Input: part model. Units: mm. Frame: model coordinates. Face numbers are marked on the shaded views. Give positions to 0.01 mm unless a question says otherwise; leave off trailing zeros. Order: outer loops, then holes, each group sorted by start corner. A loop starts at its lowest first (then second) coordinate and runs counter-clockwise, first axis right, second up. Notation, with made-up numbers: (74, 56) -> (125, 56) arc R30 cw to (125, 92) -> close; hole circle Ø4 at (67, 86.5). An arc over 180 degrees is marked (long way). Use a Markdown table: item, result. Add a question column.
from build123d import *

# Parameters (mm, degrees)
F0_R     = 14.2875
F1_DEPTH = 25.4
F2_DEPTH = 50.8


with BuildPart() as f1:
    # F0 (on Front) → F1 (new body)
    with BuildSketch(Plane.XZ):
        with BuildLine():
            Line((9.5121844836, 26.9452959039), (0, 28.575))
            ThreePointArc((0, 28.575), (-28.575, 0), (0, -28.575))
            Line((0, -28.575), (9.5121844836, -26.9452959039))
            ThreePointArc((9.5121844836, -26.9452959039), (23.3274655355, -16.5033322905), (28.575, 0))
            ThreePointArc((28.575, 0), (23.3274655355, 16.5033322905), (9.5121844836, 26.9452959039))
        make_face()
        with BuildLine():
            ThreePointArc((-14.6329037383, 4.7625), (0, 15.3884137605), (14.6329037383, 4.7625))
            Line((14.6329037383, 4.7625), (19.05, 4.7625))
            Line((19.05, 4.7625), (19.05, -4.7625))
            Line((19.05, -4.7625), (14.6329037383, -4.7625))
            ThreePointArc((14.6329037383, -4.7625), (0, -15.3884137605), (-14.6329037383, -4.7625))
            Line((-14.6329037383, -4.7625), (-19.05, -4.7625))
            Line((-19.05, -4.7625), (-19.05, 4.7625))
            Line((-19.05, 4.7625), (-14.6329037383, 4.7625))
        make_face(mode=Mode.SUBTRACT)
        with BuildLine():
            Line((57.1919272622, 18.7764181619), (9.5121844836, 26.9452959039))
            ThreePointArc((9.5121844836, 26.9452959039), (23.3274655355, 16.5033322905), (28.575, 0))
            ThreePointArc((28.575, 0), (23.3274655355, -16.5033322905), (9.5121844836, -26.9452959039))
            Line((9.5121844836, -26.9452959039), (57.1919272622, -18.7764181619))
            ThreePointArc((57.1919272622, -18.7764181619), (34.925, 0), (57.1919272622, 18.7764181619))
        make_face()
        with BuildLine():
            ThreePointArc((73.025, 0), (68.5383952831, 12.2804730295), (57.1919272622, 18.7764181619))
            ThreePointArc((57.1919272622, 18.7764181619), (34.925, 0), (57.1919272622, -18.7764181619))
            ThreePointArc((57.1919272622, -18.7764181619), (68.5383952831, -12.2804730295), (73.025, 0))
        make_face()
        with Locations((53.975, 0)):
            Circle(F0_R, mode=Mode.SUBTRACT)
        with BuildLine():
            ThreePointArc((-14.6329037383, -4.7625), (-15.3884137605, 0), (-14.6329037383, 4.7625))
            Line((-14.6329037383, 4.7625), (-19.05, 4.7625))
            Line((-19.05, 4.7625), (-19.05, -4.7625))
            Line((-19.05, -4.7625), (-14.6329037383, -4.7625))
        make_face()
    extrude(amount=F1_DEPTH)

    # F0 (on Front) → F2 (join)
    with BuildSketch(Plane.XZ):
        with BuildLine():
            Line((9.5121844836, 26.9452959039), (0, 28.575))
            ThreePointArc((0, 28.575), (-28.575, 0), (0, -28.575))
            Line((0, -28.575), (9.5121844836, -26.9452959039))
            ThreePointArc((9.5121844836, -26.9452959039), (23.3274655355, -16.5033322905), (28.575, 0))
            ThreePointArc((28.575, 0), (23.3274655355, 16.5033322905), (9.5121844836, 26.9452959039))
        make_face()
        with BuildLine():
            ThreePointArc((-14.6329037383, 4.7625), (0, 15.3884137605), (14.6329037383, 4.7625))
            Line((14.6329037383, 4.7625), (19.05, 4.7625))
            Line((19.05, 4.7625), (19.05, -4.7625))
            Line((19.05, -4.7625), (14.6329037383, -4.7625))
            ThreePointArc((14.6329037383, -4.7625), (0, -15.3884137605), (-14.6329037383, -4.7625))
            Line((-14.6329037383, -4.7625), (-19.05, -4.7625))
            Line((-19.05, -4.7625), (-19.05, 4.7625))
            Line((-19.05, 4.7625), (-14.6329037383, 4.7625))
        make_face(mode=Mode.SUBTRACT)
        with BuildLine():
            ThreePointArc((-14.6329037383, -4.7625), (-15.3884137605, 0), (-14.6329037383, 4.7625))
            Line((-14.6329037383, 4.7625), (-19.05, 4.7625))
            Line((-19.05, 4.7625), (-19.05, -4.7625))
            Line((-19.05, -4.7625), (-14.6329037383, -4.7625))
        make_face()
    extrude(amount=F2_DEPTH)


solid = f1.part
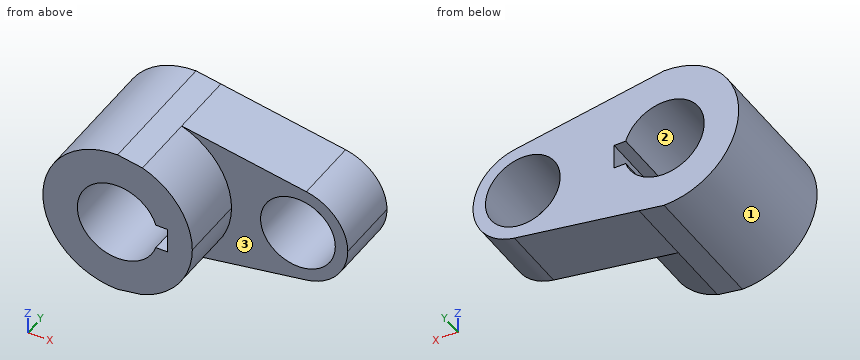
Q1. Section query B-B (z = -7.5). Return loops of the section in (x, y), plus the area to 3 significant figures.
Q2. First-contact query: pin 1 (3.5 mm diameter, centred on x = 16.5, y = -33, fed in from +Z); pin 2 (10.5 mm diameter, centred on y = -13.5, z = -1.5, fed in from -X) (3 decimals); pin 3 (3 mm diameter, centred on x = 7.5, z = -11.5, fed in from +Y); pin 4 (16 mm diameter, centred on x = 46.5, z = 7, fed in from -Y). Flat tips, straight axial feed; report the tip coordinate or a pass-through.
Q3. Ray query, line 1 (X direction, y = -10.5, z = -8.5); line 2 (X direction, y = -11.5, z = -3.5); line 3 (Y direction, x = 44.5, z = -14). Return the intervals inside material, ascending.
Q4. Section query D-D (x = 52). Return loops of the section in (y, z).
Q5. Draft query along X for the marked faces 1, 2 and 3. Return one class per face: +X half, -X half, draft (parallel to the pull), parting line (faces both ways), or undercut.
Q6. Section query C-C (y = -12.5). Give the number of separate pieces and of enclosed holes in the cut face, plus the area to 3 significant figures.
Solution:
| question | item | result |
|---|---|---|
| 1 | outline | (-27.57, -50.8) -> (-13.44, -50.8) -> (-13.44, 0) -> (-27.57, 0) -> close; (13.44, -50.8) -> (27.57, -50.8) -> (27.57, -25.4) -> (41.81, -25.4) -> (41.81, 0) -> (13.44, 0) -> close; (66.14, -25.4) -> (71.49, -25.4) -> (71.49, 0) -> (66.14, 0) -> close |
| 1 | area | 1,930 mm² |
| 2 | pin 1 | stops at z = 24.47 |
| 2 | pin 2 | stops at x = -28.575 |
| 2 | pin 3 | passes through |
| 2 | pin 4 | stops at y = -25.4 |
| 3 | line 1 | x = -27.28 to -12.83, 12.83 to 42.49, 65.46 to 71.02 |
| 3 | line 2 | x = -28.36 to -14.99, 19.05 to 40.12, 67.83 to 72.7 |
| 3 | line 3 | y = -25.4 to 0 |
| 4 | outline | (-25.4, -19.67) -> (0, -19.67) -> (0, -14.15) -> (-25.4, -14.15) -> close; (-25.4, 14.15) -> (0, 14.15) -> (0, 19.67) -> (-25.4, 19.67) -> close |
| 5 | face 1 | -X half |
| 5 | face 2 | undercut |
| 5 | face 3 | draft |
| 6 | separate pieces | 1 |
| 6 | enclosed holes | 2 |
| 6 | area | 3,020 mm² |
